Autodesk Inventor part; units mm, degrees
ref_plane "YZ Plane" through (0, 0, 0) normal (1, 0, 0) x (0, 1, 0)
ref_plane "XZ Plane" through (0, 0, 0) normal (0, 1, 0) x (-1, 0, 0)
ref_plane "XY Plane" through (0, 0, 0) normal (0, 0, 1) x (1, 0, 0)
sketch "Sketch1" plane through (0, 0, 0) normal (0, 1, 0) x (-1, 0, 0)
  line L0 (-10.5, 65.5) -> (-10.5, -65.5)
  line L1 (-10.5, 65.5) -> (-7.5, 65.5)
  line L2 (-10.5, -65.5) -> (-7.5, -65.5)
  arc A0 (-7.5, -65.5) -> (-7.5, 65.5) centre (-117.6736, 0) ccw
  line L3 (-7.5, 65.5) -> (-10.5, 65.5)
  line L4 (-10.5, 65.5) -> (-10.5, -65.5)
  line L5 (-10.5, -65.5) -> (-7.5, -65.5)
  line L6 (-10.5, -65.5) -> (-10.5, 65.5)
  line L7 (-10.5, -65.5) -> (-10.5, -30.5)
  line L8 (-10.5, 65.5) -> (-10.5, 30.15)
  line L9 (-10.5, 30.5) -> (-10.5, -30.5)
  line L10 (-10.5, 30.5) -> (-10.5, -30.5)
  circle A1 centre (-0.5, -30.5) radius 1.5
  line L11 (-0.5, -30.5) -> (-10.5, -30.5)
  line L12 (-10.5, -30.5) -> (-10.5, 30.15)
  line L13 (-10.5, 30.15) -> (-0.5, 30.15)
  circle A2 centre (-0.5, 30.15) radius 1.5
  point P0 (0, 0)
  dimension "d2" = 3
  dimension "d3" = 3
  dimension "d13" = 35
  dimension "d14" = 35.35
  dimension "d17" = 3
  dimension "d21" = 3
extrude "Extrusion1" add sketch "Sketch1" along normal blind 2 contours A2 | A1 | L1 A0 L2 L0
extrude "Extrusion3" cut sketch "Sketch1" along normal blind 2 contours A2 | A1
properties part number "naraznik_kryt"
Check sheet for the modelled part. Datum: model origin and axes. Units: mm. Round coordinates to 2 decimals unless told otherwise and drop trailing zeros. Write each loop counter-clockwise with the first axis right and the second up, starting at its lowest first coordinate (ties: lowest second). Pieces come first, ordered by that corner, then holes. Notation, with made-up numbers: M -12,-14.75 L -6,-14.75 A20 ccw -6,23.25 Z; hole C -14.5,-35 d7. An arc over 180 degrees is marked long. Write item = value, one per line. Start each with the question number.
1. Release check for a two-part mould opening along X. For faces 1 (the flat face through (10.5, 1, 1)), 2 (the flat face through (9, 1, -65.5)), 3 (the cylindrical face through (0.695, 0.986, -31.987)) record: pulls with the +X half, pulls with the -X half, needs draft (parallel to the pull), parting line crosses it, or undercut.
2. Section check C-C, the plane x = 0.5. Record the cut outline in (y, z).
3. Gauge pin test, flat ends, axial feed: pin 1 (4 mm diameter, centred on x = -3.5, z = -42.5, fed in from -Y); pin 2 (1 mm diameter, centred on x = -0.5, y = 1.5, fed in from -Z); pin 3 (1 mm diameter, centred on y = 0.5, z = 6, fed in from -X). Record the tip position at first contact, or that the pin passes through.
4. Section check B-B, the plane y = 0.8. Record the cut outline in (x, z), then the cut area to 3 significant figures.
5. Section check D-D, the plane z = 20. Record the cut outline in (x, y), then the cut area to 3 significant figures.
6. Scan lines: line 1 (Z direction, x = 0.5, y = 1); line 2 (Z direction, x = 1.5, y = 0.35); line 3 (X direction, y = 0.55, z = -30.5). Record each from-to range of solid material in increasing order. Write a range as [from, to].
7. Section check A-A, the plane z = -30.5. Record the cut outline in (x, y).
Results found:
q1.face_1 = pulls with the +X half
q1.face_2 = needs draft
q1.face_3 = undercut
q2.outline = M 0,-51.95 L 2,-51.95 L 2,-32 L 0,-32 Z; M 0,-29 L 2,-29 L 2,28.65 L 0,28.65 Z; M 0,31.65 L 2,31.65 L 2,51.95 L 0,51.95 Z
q3.pin_1 = 0
q3.pin_2 = -50.81
q3.pin_3 = -10.38
q4.outline = M 7.5,-65.5 L 10.5,-65.5 L 10.5,65.5 L 7.5,65.5 A128.17 ccw Z; hole C 0.5,-30.5 d3; hole C 0.5,30.15 d3
q4.area = 1,970 mm^2
q5.outline = M -8.93,0 L 10.5,0 L 10.5,2 L -8.93,2 Z
q5.area = 38.9 mm^2
q6.line_1 = [-51.95, -32], [-29, 28.65], [31.65, 51.95]
q6.line_2 = [-54.15, -31.62], [-29.38, 29.03], [31.27, 54.15]
q6.line_3 = [-6.82, -1], [2, 10.5]
q7.outline = M -6.82,0 L -1,0 L -1,2 L -6.82,2 Z; M 2,0 L 10.5,0 L 10.5,2 L 2,2 Z
